Geometry: final body of the model. Coordinates: model frame, mm. A direction names the side the tool comes from. Give positions to 0.01 mm unless a question says otherwise; leave off trailing zeros. Write each loop counter-clockwise with the first axis right and the second up, starting at its lowest first coordinate (ties: lowest second). Pieces come first, ordered by that corner, then holes. Notation, with made-up numbers: M -34,12 L -4,12 A21 cw -4,46 Z; hole C 60.5,64 d6. An arc over 180 degrees is marked long. Use a Markdown table: item, result. Add a question column.
(1) Cut plane D-D (z = -16.75). Output: boundary loops of the cut face in (x, y).
(2) Draft query along Z for faces 4 (the flat face through (-1, 8, 30)), 5 (the flat face through (84.85, 8, 0)), 6 (the cylindrical face through (-15.9, 7.9, -19.5)). Return one class per face: released by +Z, released by -Z, zero draft, split by the parting line, or undercut.
(3) Cut plane A-A (z = 0). Output: boundary loops of the cut face in (x, y), plus the area to 3 significant figures.
(4) Material intervals for L1, parallel to X at y = 32.5, z = -11; L2, parallel to X at y = 6.5, z = -16.75; L3, parallel to Y at x = 69.5, z = 0, sorted ascending.
(5) Reachability of faces 1 (the flat face through (72, 20, 24.175)), 2 (the flat face through (-80.85, 34, 0)), 3 (the flat face through (79.67, 34, 0)) from +Z, -Z, +X, -X, +Y, -Y: full face, straight path, thin tool, end or side. Return the list, or none.
(6) Cut plane B-B (x = 43.9). Output: boundary loops of the cut face in (y, z), plus the area to 3 significant figures.
(7) Pin query (flat end, axial travel): pin 1 Ø22 at (y, z) = (31, 3) entering from -X; pin 2 Ø5 at (x, z) = (4.5, 18.5) entering from +Y; pin 3 Ø4 at (x, y) = (-42, 21.5) entering from +Z (3 decimals). Return the tip coordinate at first contact, or that it passes through.
(8) Cut plane C-C (y = 18). Output: boundary loops of the cut face in (x, z) (3 decimals).
```python
from build123d import *

# Parameters (mm, degrees)
SKETCH1_W           = 169.7
SKETCH1_H           = 60
SKETCH1_R           = 2.75
BOSS_EXTRUDE1_DEPTH = 16
BOSS_EXTRUDE2_START = -5.18
SKETCH2_W           = 48.35
SKETCH2_H           = 8.5
SKETCH2_W_2         = 26.35
SKETCH2_H_2         = 35.9
SKETCH2_R           = 7.95
BOSS_EXTRUDE2_DEPTH = 16
BOSS_EXTRUDE3_START = -149.7
SKETCH2_3_W         = 48.35
SKETCH2_3_H         = 8.5
SKETCH2_3_W_2       = 26.35
SKETCH2_3_H_2       = 35.9
SKETCH2_3_R         = 7.95
BOSS_EXTRUDE3_DEPTH = 16
LPATTERN1_COUNT     = 2
LPATTERN1_PITCH     = 30


with BuildPart() as part:
    # Sketch1 → Boss-Extrude1 (new body)
    with BuildSketch(Plane(origin=(0, 0, 0), x_dir=(1, 0, 0), z_dir=(0, 1, 0))):
        Rectangle(SKETCH1_W, SKETCH1_H)
        with Locations(Location((-16, -16.75, 0), (0, 0, 270))):
            Circle(SKETCH1_R, mode=Mode.SUBTRACT)
        with Locations(Location((43.9, -16.75, 0), (0, 0, 270))):
            Circle(SKETCH1_R, mode=Mode.SUBTRACT)
        with Locations(Location((43.9, 16.75, 0), (0, 0, 270))):
            Circle(SKETCH1_R, mode=Mode.SUBTRACT)
        with Locations(Location((-16, 16.75, 0), (0, 0, 270))):
            Circle(SKETCH1_R, mode=Mode.SUBTRACT)
    extrude(amount=BOSS_EXTRUDE1_DEPTH)

    # Sketch2 → Boss-Extrude2 (add)
    # profile 1 of 2: a face of its own
    with BuildSketch(Plane(origin=(84.85, 0, 0), x_dir=(0, 0, -1), z_dir=(1, 0, 0)).offset(BOSS_EXTRUDE2_START)):
        with Locations((0, 20.25)):
            Rectangle(SKETCH2_W, SKETCH2_H)
    # profile 2 of 2: a face of its own
    with BuildSketch(Plane(origin=(84.85, 0, 0), x_dir=(0, 0, -1), z_dir=(1, 0, 0)).offset(BOSS_EXTRUDE2_START)):
        with Locations((0, 42.45)):
            Rectangle(SKETCH2_W_2, SKETCH2_H_2)
        with Locations((0, 43.25)):
            Circle(SKETCH2_R, mode=Mode.SUBTRACT)
    extrude(amount=-BOSS_EXTRUDE2_DEPTH)

    # Sketch2<3> → Boss-Extrude3 (add)
    # profile 1 of 2: a face of its own
    with BuildSketch(Plane(origin=(84.85, 0, 0), x_dir=(0, 0, -1), z_dir=(1, 0, 0)).offset(BOSS_EXTRUDE3_START)):
        with Locations((0, 20.25)):
            Rectangle(SKETCH2_3_W, SKETCH2_3_H)
    # profile 2 of 2: a face of its own
    with BuildSketch(Plane(origin=(84.85, 0, 0), x_dir=(0, 0, -1), z_dir=(1, 0, 0)).offset(BOSS_EXTRUDE3_START)):
        with Locations((0, 42.45)):
            Rectangle(SKETCH2_3_W_2, SKETCH2_3_H_2)
        with Locations((0, 43.25)):
            Circle(SKETCH2_3_R, mode=Mode.SUBTRACT)
    boss_extrude3 = extrude(amount=-BOSS_EXTRUDE3_DEPTH)

    # LPattern1: Boss-Extrude3 ×2
    with Locations(*[(i * LPATTERN1_PITCH, 0, 0) for i in range(1, LPATTERN1_COUNT)]):
        add(boss_extrude3)


solid = part.part
```
Answer list:
| question | item | result |
|---|---|---|
| 1 | outline | M -84.85,0 L -18.75,0 L -18.75,16 L -34.85,16 L -34.85,24.5 L -50.85,24.5 L -50.85,16 L -64.85,16 L -64.85,24.5 L -80.85,24.5 L -80.85,16 L -84.85,16 Z; M -13.25,0 L 41.15,0 L 41.15,16 L -13.25,16 Z; M 46.65,0 L 84.85,0 L 84.85,16 L 79.67,16 L 79.67,24.5 L 63.67,24.5 L 63.67,16 L 46.65,16 Z |
| 2 | face 4 | released by +Z |
| 2 | face 5 | zero draft |
| 2 | face 6 | undercut |
| 3 | outline | M -84.85,0 L 84.85,0 L 84.85,16 L 79.67,16 L 79.67,35.3 L 63.67,35.3 L 63.67,16 L -34.85,16 L -34.85,35.3 L -50.85,35.3 L -50.85,16 L -64.85,16 L -64.85,35.3 L -80.85,35.3 L -80.85,16 L -84.85,16 Z; M -80.85,51.2 L -64.85,51.2 L -64.85,60.4 L -80.85,60.4 Z; M -50.85,51.2 L -34.85,51.2 L -34.85,60.4 L -50.85,60.4 Z; M 63.67,51.2 L 79.67,51.2 L 79.67,60.4 L 63.67,60.4 Z |
| 3 | area | 4,080 mm² |
| 4 | L1 | -80.85 to -64.85, -50.85 to -34.85, 63.67 to 79.67 |
| 4 | L2 | -84.85 to -18.75, -13.25 to 41.15, 46.65 to 84.85 |
| 4 | L3 | 0 to 35.3, 51.2 to 60.4 |
| 5 | face 1 | +Z, +X, -X, +Y |
| 5 | face 2 | +Z, -Z, -X, +Y |
| 5 | face 3 | +Z, -Z, +X, +Y |
| 6 | outline | M 0,-30 L 16,-30 L 16,-19.5 L 0,-19.5 Z; M 0,-14 L 16,-14 L 16,14 L 0,14 Z; M 0,19.5 L 16,19.5 L 16,30 L 0,30 Z |
| 6 | area | 784 mm² |
| 7 | pin 1 | x = -80.85 |
| 7 | pin 2 | y = 16 |
| 7 | pin 3 | z = 24.175 |
| 8 | outline | M -80.85,-24.175 L -64.85,-24.175 L -64.85,24.175 L -80.85,24.175 Z; M -50.85,-24.175 L -34.85,-24.175 L -34.85,24.175 L -50.85,24.175 Z; M 63.67,-24.175 L 79.67,-24.175 L 79.67,24.175 L 63.67,24.175 Z |
